from build123d import *

# Parameters (mm, degrees)
ESQUISSE1_W                    = 203.5
ESQUISSE1_H                    = 35
BOSS_EXTRU_1_DEPTH             = 1
CONG_1_R                       = 9
BOSS_EXTRU_2_START             = 8.5
BOSS_EXTRU_2_DEPTH             = 8.5
BOSS_EXTRU_3_DEPTH             = 1
CONG_2_R                       = 4
CONG_3_R                       = 0.5
BOSS_EXTRU_4_START             = 91.75
BOSS_EXTRU_4_DEPTH             = 20
ESQUISSE8_W                    = 20
ESQUISSE8_H                    = 120.5
BOSS_EXTRU_5_DEPTH             = 6.5
ESQUISSE9_R                    = 4.25
BOSS_EXTRU_6_DEPTH             = 20
BOSS_EXTRU_10_START            = 51.75
BOSS_EXTRU_10_DEPTH            = 100
BOSS_EXTRU_10_START_2          = 91.75
BOSS_EXTRU_10_2_OUTLINE_W      = 12.5
BOSS_EXTRU_10_2_OUTLINE_H      = 25.5
BOSS_EXTRU_10_2_DEPTH          = 20
ESQUISSE21_W                   = 25
ESQUISSE21_H                   = 1
BOSS_EXTRU_11_DEPTH            = 100
ENL_V_MAT_EXTRU_2_DEPTH        = 4
R_P_TITION_LIN_AIRE2_COUNT     = 2
R_P_TITION_LIN_AIRE2_PITCH     = 8
ENL_V_START                    = -20
ESQUISSE12_R                   = 1.6
ENL_V_MAT_EXTRU_4_DEPTH        = 20
BOSS_EXTRU_7_START             = 11
BOSS_EXTRU_7_DEPTH             = 18
ESQUISSE15_W                   = 18
ESQUISSE15_H                   = 5
BOSS_EXTRU_8_DEPTH             = 12
ENL_V_MAT_EXTRU_5_REACH        = 260.26
ESQUISSE16_R                   = 1
ESQUISSE17_W                   = 4
ESQUISSE17_H                   = 23.5
BOSS_EXTRU_9_DEPTH             = 2
R_P_TITION_LIN_AIRE1_COUNT     = 2
R_P_TITION_LIN_AIRE1_PITCH     = 7
R_P_TITION_LIN_AIRE1_COL_COUNT = 2
R_P_TITION_LIN_AIRE1_COL_PITCH = 7
ENL_V_MAT_EXTRU_6_REACH        = 266.365
ESQUISSE18_W                   = 6.5
ESQUISSE18_H                   = 8.5


# Read off the part's stored shape, not the designer's step: Boss.-Extru.4, Boss.-Extru.10, Boss.-Extru.7
with BuildPart() as part:
    # Esquisse1 → Boss.-Extru.1 (new body)
    with BuildSketch(Plane.XY):
        with Locations((101.75, 17.5)):
            Rectangle(ESQUISSE1_W, ESQUISSE1_H)
    extrude(amount=BOSS_EXTRU_1_DEPTH)

    # Congé1
    cong_1_edges = [part.edges().sort_by_distance(p)[0] for p in [
        (203.5, 0, 0.5),
        (0, 0, 0.5),
    ]]
    fillet(cong_1_edges, radius=CONG_1_R)

    # Esquisse3 → Boss.-Extru.2 (add)
    with BuildSketch(Plane.XY.offset(1).offset(BOSS_EXTRU_2_START)):
        with BuildLine():
            Line((1.5, 33.5), (1.5, 35))
            Line((1.5, 35), (0, 35))
            Line((0, 35), (0, 9))
            ThreePointArc((0, 9), (2.636038969, 2.636038969), (9, 0))
            Line((9, 0), (194.5, 0))
            ThreePointArc((194.5, 0), (200.863961031, 2.636038969), (203.5, 9))
            Line((203.5, 9), (203.5, 35))
            Line((203.5, 35), (202, 35))
            Line((202, 35), (202, 33.5))
            Line((202, 33.5), (202, 9))
            ThreePointArc((202, 9), (199.803300859, 3.696699141), (194.5, 1.5))
            Line((194.5, 1.5), (9, 1.5))
            ThreePointArc((9, 1.5), (3.696699141, 3.696699141), (1.5, 9))
            Line((1.5, 9), (1.5, 33.5))
        make_face()
    extrude(amount=-BOSS_EXTRU_2_DEPTH)

    # Esquisse4 → Boss.-Extru.3 (add)
    with BuildSketch(Plane.XY.offset(9.5)):
        with BuildLine():
            Line((6.5, 35), (6.5, 9))
            ThreePointArc((6.5, 9), (7.232233047, 7.232233047), (9, 6.5))
            Line((9, 6.5), (194.5, 6.5))
            ThreePointArc((194.5, 6.5), (196.267766953, 7.232233047), (197, 9))
            Line((197, 9), (197, 35))
            Line((197, 35), (203.5, 35))
            Line((203.5, 35), (203.5, 9))
            ThreePointArc((203.5, 9), (200.863961031, 2.636038969), (194.5, 0))
            Line((194.5, 0), (9, 0))
            ThreePointArc((9, 0), (2.636038969, 2.636038969), (0, 9))
            Line((0, 9), (0, 35))
            Line((0, 35), (6.5, 35))
        make_face()
    extrude(amount=-BOSS_EXTRU_3_DEPTH)

    # Congé2
    cong_2_edges = [part.edges().sort_by_distance(p)[0] for p in [
        (203.5, 22, 0),
        (101.75, 0, 0),
        (2.636038969, 2.636038969, 0),
        (200.863961031, 2.636038969, 0),
        (3.696699141, 3.696699141, 1),
        (101.75, 1.5, 1),
        (199.803300859, 3.696699141, 1),
        (202, 22, 1),
        (1.5, 22, 1),
        (0, 22, 0),
    ]]
    fillet(cong_2_edges, radius=CONG_2_R)

    # Congé3
    cong_3_edges = [part.edges().sort_by_distance(p)[0] for p in [
        (101.75, 1.5, 8.5),
        (1.5, 22, 8.5),
        (3.696699141, 3.696699141, 8.5),
        (199.803300859, 3.696699141, 8.5),
        (202, 22, 8.5),
    ]]
    fillet(cong_3_edges, radius=CONG_3_R)

    # Boss.-Extru.4 outline → Boss.-Extru.4 (add)
    with BuildSketch(Plane.YZ.offset(BOSS_EXTRU_4_START)):
        with BuildLine():
            Line((-2, 130), (-2, 0))
            Line((-2, 0), (4, 0))
            ThreePointArc((4, 0), (1.171572875, 1.171572875), (0, 4))
            Line((0, 4), (0, 130))
            Line((0, 130), (-2, 130))
        make_face()
    extrude(amount=BOSS_EXTRU_4_DEPTH)

    # Esquisse8 → Boss.-Extru.5 (add)
    with BuildSketch(Plane(origin=(0, 0, 0), x_dir=(1, 0, 0), z_dir=(0, 1, 0))):
        with Locations((101.75, -69.75)):
            Rectangle(ESQUISSE8_W, ESQUISSE8_H)
    extrude(amount=BOSS_EXTRU_5_DEPTH)

    # Esquisse9 → Boss.-Extru.6 (add)
    with BuildSketch(Plane.ZY.offset(-91.75)):
        with Locations((130, 2.25)):
            Circle(ESQUISSE9_R)
    extrude(amount=-BOSS_EXTRU_6_DEPTH)

    # Boss.-Extru.10 outline → Boss.-Extru.10 (add)
    with BuildSketch(Plane.YZ.offset(BOSS_EXTRU_10_START)):
        with BuildLine():
            Line((0, 4), (0, 9.5))
            Line((0, 9.5), (-14.5, 9.5))
            Line((-14.5, 9.5), (-14.5, 0))
            Line((-14.5, 0), (4, 0))
            ThreePointArc((4, 0), (1.171572875, 1.171572875), (0, 4))
        make_face()
    extrude(amount=BOSS_EXTRU_10_DEPTH)

    # Boss.-Extru.10 2 outline → Boss.-Extru.10 2 (add)
    with BuildSketch(Plane.YZ.offset(BOSS_EXTRU_10_START_2)):
        with Locations((-8.25, 22.25)):
            Rectangle(BOSS_EXTRU_10_2_OUTLINE_W, BOSS_EXTRU_10_2_OUTLINE_H)
    extrude(amount=BOSS_EXTRU_10_2_DEPTH)

    # Esquisse21 → Boss.-Extru.11 (add)
    with BuildSketch(Plane(origin=(0, 35, 0), x_dir=(1, 0, 0), z_dir=(0, 1, 0))):
        with Locations((101.75, -0.5)):
            Rectangle(ESQUISSE21_W, ESQUISSE21_H)
    extrude(amount=BOSS_EXTRU_11_DEPTH)

    # Esquisse10 → Enlèv. mat.-Extru.2 (cut)
    with BuildSketch(Plane(origin=(95.75, 0, 0), x_dir=(0, 0, -1), z_dir=(1, 0, 0))):
        with BuildLine():
            Line((-125.75, 2.25), (-125.75, 6.5))
            Line((-125.75, 6.5), (-130, 6.5))
            ThreePointArc((-130, 6.5), (-133.00520382, -0.75520382), (-125.75, 2.25))
        make_face()
    enl_v_mat_extru_2 = extrude(amount=ENL_V_MAT_EXTRU_2_DEPTH, mode=Mode.SUBTRACT)

    # Répétition linéaire2: Enlèv. mat.-Extru.2 ×2
    with Locations(*[(i * R_P_TITION_LIN_AIRE2_PITCH, 0, 0) for i in range(1, R_P_TITION_LIN_AIRE2_COUNT)]):
        add(enl_v_mat_extru_2, mode=Mode.SUBTRACT)

    # Esquisse12 → Enlèv. mat.-Extru.4 (cut)
    with BuildSketch(Plane.ZY.offset(-91.75).offset(ENL_V_START)):
        with Locations((130, 2.25)):
            Circle(ESQUISSE12_R)
    extrude(amount=ENL_V_MAT_EXTRU_4_DEPTH, mode=Mode.SUBTRACT)

    # Boss.-Extru.7 outline → Boss.-Extru.7 (add)
    with BuildSketch(Plane.YZ.offset(BOSS_EXTRU_7_START)):
        with BuildLine():
            Line((0, 33), (-2, 33))
            Line((-2, 33), (-2, 0))
            Line((-2, 0), (4, 0))
            ThreePointArc((4, 0), (1.171572875, 1.171572875), (0, 4))
            Line((0, 4), (0, 33))
        make_face()
    extrude(amount=BOSS_EXTRU_7_DEPTH)

    # Esquisse15 → Boss.-Extru.8 (add)
    with BuildSketch(Plane.XZ.offset(2)):
        with Locations((20, 2.5)):
            Rectangle(ESQUISSE15_W, ESQUISSE15_H)
        with Locations((20, 30.5)):
            Rectangle(ESQUISSE15_W, ESQUISSE15_H)
    extrude(amount=BOSS_EXTRU_8_DEPTH)

    # Esquisse16 → Enlèv. mat.-Extru.5 (cut, up to next)
    with BuildSketch(Plane(origin=(29, 0, 0), x_dir=(0, 0, -1), z_dir=(1, 0, 0)), mode=Mode.PRIVATE) as enl_v_mat_extru_5_sk1:
        with Locations((-30.5, -8)):
            Circle(ESQUISSE16_R)
    enl_v_mat_extru_5_tool1 = extrude(enl_v_mat_extru_5_sk1.sketch, amount=-ENL_V_MAT_EXTRU_5_REACH, mode=Mode.PRIVATE) & part.part
    # Esquisse16 → Enlèv. mat.-Extru.5 (cut, up to next)
    with BuildSketch(Plane(origin=(29, 0, 0), x_dir=(0, 0, -1), z_dir=(1, 0, 0)), mode=Mode.PRIVATE) as enl_v_mat_extru_5_sk2:
        with Locations((-2.5, -8)):
            Circle(ESQUISSE16_R)
    enl_v_mat_extru_5_tool2 = extrude(enl_v_mat_extru_5_sk2.sketch, amount=-ENL_V_MAT_EXTRU_5_REACH, mode=Mode.PRIVATE) & part.part
    add(enl_v_mat_extru_5_tool1.solids().sort_by_distance((29, -8, 30.5))[0], mode=Mode.SUBTRACT)
    add(enl_v_mat_extru_5_tool2.solids().sort_by_distance((29, -8, 2.5))[0], mode=Mode.SUBTRACT)

    # Esquisse17 → Boss.-Extru.9 (add)
    with BuildSketch(Plane(origin=(0, 0, 0), x_dir=(1, 0, 0), z_dir=(0, 1, 0))):
        with Locations((20, -21.25)):
            Rectangle(ESQUISSE17_W, ESQUISSE17_H)
    boss_extru_9 = extrude(amount=BOSS_EXTRU_9_DEPTH)

    # Répétition linéaire1: Boss.-Extru.9 ×2
    with Locations(*[(i * R_P_TITION_LIN_AIRE1_PITCH, 0, 0) for i in range(1, R_P_TITION_LIN_AIRE1_COUNT)]):
        add(boss_extru_9)

    # Répétition linéaire1 col: Boss.-Extru.9 ×2
    with Locations(*[(-i * R_P_TITION_LIN_AIRE1_COL_PITCH, 0, 0) for i in range(1, R_P_TITION_LIN_AIRE1_COL_COUNT)]):
        add(boss_extru_9)

    # Esquisse18 → Enlèv. mat.-Extru.6 (cut, up to next)
    with BuildSketch(Plane.XY.offset(33), mode=Mode.PRIVATE) as enl_v_mat_extru_6_sk1:
        with Locations((14.25, -9.75)):
            Rectangle(ESQUISSE18_W, ESQUISSE18_H)
    enl_v_mat_extru_6_tool1 = extrude(enl_v_mat_extru_6_sk1.sketch, amount=-ENL_V_MAT_EXTRU_6_REACH, mode=Mode.PRIVATE) & part.part
    add(enl_v_mat_extru_6_tool1.solids().sort_by_distance((14.25, -9.75, 33))[0], mode=Mode.SUBTRACT)


solid = part.part
Check sheet for the modelled part. Datum: model origin and axes. Units: mm. A direction names the side the tool comes from. Coordinates: 2 decimals unless noted, no trailing zeros. Loops run counter-clockwise (first coordinate to the right, second up) from the corner with the lowest first, then second, coordinate; pieces in that order, holes last. Notation, with made-up numbers: (72, -16.75) -> (81, -16.75) arc R29 cw to (81, 20.25) -> close; hole circle Ø11 at (70.25, 79.25). An arc over 180 degrees is marked (long way). Write item = value, one per line. Start each with the question number.
1. Section check A-A on x = 72. Record the cut outline in (y, z), then the cut area to 3 significant figures.
2. Draft check along X on faces 4 (the cylindrical face through (199.861, 3.755, 6.521)), 5 (the flat face through (151, 1, 9.5)), 6 (the flat face through (11, -1.7, 14.1)). Enter one of: released by +X, released by -X, zero draft, split by the parting line, or undercut.
3. Material ranges on line 1 (Z direction, x = 101, y = 2); line 2 (Z direction, x = 102.65, y = 2.25); line 3 (Y direction, x = 101.1, z = 130), recorded low to high.
4. Tool access check on faces 1 (the flat face through (14, -5.5, 31)), 2 (the flat face through (95.75, 2, 128)), 3 (the flat face through (23, -14, 31)). Record the directions out of +Z, -Z, +X, -X, +Y, -Y that give a thin tool (end or side, any length) a straight path to the whole face; none if there is none.
5. Section check B-B on y = 19. Record the cut outline in (x, z), then the cut area to 3 significant figures.
6. Depth check by flat-ended pin: P1, Ø2.5, axis at y = 4.5, z = 131.5, coming from the -X side; P2, Ø20, axis at x = 22, z = 14, coming from the -Y side; P3, Ø13, axis at x = 18, y = -8, coming from the +Z side; P4, Ø5, axis at y = 10.5, z = 62, coming from the -X side. Enter the tip coordinate at first touch or a pass-through.
7. Section check C-C on z = 44.5. Record the cut outline in (x, y), then the cut area to 3 significant figures.
8. Section check D-D on y = 41.5. Record the cut outline in (x, z).
Responses:
q1.outline = (-14.5, 0) -> (35, 0) -> (35, 1) -> (5.5, 1) arc R4 cw to (1.5, 5) -> (1.5, 8) arc R0.5 cw to (2, 8.5) -> (6.5, 8.5) -> (6.5, 9.5) -> (-14.5, 9.5) -> close
q1.area = 194 mm2
q2.face_4 = undercut
q2.face_5 = zero draft
q2.face_6 = released by -X
q3.line_1 = 0 to 3.06, 8.5 to 128.42, 131.58 to 134.24
q3.line_2 = 0 to 2.67, 8.5 to 128.4, 131.6 to 134.25
q3.line_3 = -2 to 0.65, 3.85 to 6.5
q4.face_1 = +Z, -X, -Y
q4.face_2 = +Z, +Y
q4.face_3 = +Z, -Z, -X, -Y
q5.outline = (0, 4) arc R4 ccw to (4, 0) -> (199.5, 0) arc R4 ccw to (203.5, 4) -> (203.5, 9.5) -> (197, 9.5) -> (197, 8.5) -> (201.5, 8.5) arc R0.5 cw to (202, 8) -> (202, 5) arc R4 cw to (198, 1) -> (5.5, 1) arc R4 cw to (1.5, 5) -> (1.5, 8) arc R0.5 cw to (2, 8.5) -> (6.5, 8.5) -> (6.5, 9.5) -> (0, 9.5) -> close
q5.area = 239 mm2
q6.P1 = 91.75
q6.P2 = -14
q6.P3 = 33
q6.P4 = through
q7.outline = (91.75, -2) -> (111.75, -2) -> (111.75, 6.5) -> (91.75, 6.5) -> close
q7.area = 170 mm2
q8.outline = (89.25, 0) -> (114.25, 0) -> (114.25, 1) -> (89.25, 1) -> close
